Check sheet for the modelled part. Datum: model origin and axes. Units: mm. Give positions to 0.01 mm unless a question says otherwise; leave off trailing zeros. Loops run counter-clockwise (first coordinate to the right, second up) from the corner with the lowest first, then second, coordinate; pieces in that order, holes last. Notation, with made-up numbers: (-22.75, -7) - (23.25, -7) arc R25 ccw to (23.25, 7) - close; hole circle Ø7 at (28, 50). An arc over 180 degrees is marked (long way). Use CSV: the item, a comma, the result in double quotes.
from build123d import *

# Parameters (mm, degrees)
SKETCH1_R           = 0.75
SKETCH1_R_2         = 1.64
BOSS_EXTRUDE1_DEPTH = 2.3


with BuildPart() as part:
    # Sketch1 → Boss-Extrude1 (new body)
    with BuildSketch(Plane.XY):
        with BuildLine():
            Line((-16.1, -2.500431312), (-4.640508927, -3.959252063))
            ThreePointArc((-4.640508927, -3.959252063), (0, -6.1), (4.640508927, -3.959252063))
            Line((4.640508927, -3.959252063), (16.1, -2.500431312))
            ThreePointArc((16.1, -2.500431312), (18.598607316, 0.095489412), (15.90916049, 2.493137988))
            Line((15.90916049, 2.493137988), (4.649322288, 3.948898867))
            ThreePointArc((4.649322288, 3.948898867), (0, 6.1), (-4.649322288, 3.948898867))
            Line((-4.649322288, 3.948898867), (-15.90916049, 2.493137988))
            ThreePointArc((-15.90916049, 2.493137988), (-18.598607316, 0.095489412), (-16.1, -2.500431312))
        make_face()
        with Locations((-16.1, 0)):
            Circle(SKETCH1_R, mode=Mode.SUBTRACT)
        with BuildLine():
            ThreePointArc((-12.55, 0), (-13.3, -0.75), (-14.05, 0))
            ThreePointArc((-14.05, 0), (-13.3, 0.75), (-12.55, 0))
        make_face(mode=Mode.SUBTRACT)
        with BuildLine():
            ThreePointArc((-9.75, 0), (-10.5, -0.75), (-11.25, 0))
            ThreePointArc((-11.25, 0), (-10.5, 0.75), (-9.75, 0))
        make_face(mode=Mode.SUBTRACT)
        with BuildLine():
            ThreePointArc((-6.95, 0), (-7.7, -0.75), (-8.45, 0))
            ThreePointArc((-8.45, 0), (-7.7, 0.75), (-6.95, 0))
        make_face(mode=Mode.SUBTRACT)
        Circle(SKETCH1_R_2, mode=Mode.SUBTRACT)
        with BuildLine():
            ThreePointArc((8.45, 0), (7.7, -0.75), (6.95, 0))
            ThreePointArc((6.95, 0), (7.7, 0.75), (8.45, 0))
        make_face(mode=Mode.SUBTRACT)
        with BuildLine():
            ThreePointArc((11.25, 0), (10.5, -0.75), (9.75, 0))
            ThreePointArc((9.75, 0), (10.5, 0.75), (11.25, 0))
        make_face(mode=Mode.SUBTRACT)
        with BuildLine():
            ThreePointArc((14.05, 0), (13.3, -0.75), (12.55, 0))
            ThreePointArc((12.55, 0), (13.3, 0.75), (14.05, 0))
        make_face(mode=Mode.SUBTRACT)
        with Locations((16.1, 0)):
            Circle(SKETCH1_R, mode=Mode.SUBTRACT)
    extrude(amount=BOSS_EXTRUDE1_DEPTH)


solid = part.part
1. Sectioned sample at A-A, the plane x = -10.5. Record the boundary of the cut face in (y, z), and give its area (3 significant figures).
Completed:
outline,"(-3.21, 0) - (-0.75, 0) - (-0.75, 2.3) - (-3.21, 2.3) - close; (0.75, 0) - (3.19, 0) - (3.19, 2.3) - (0.75, 2.3) - close"
area,"11.3 mm²"
2. Sectioned sample at D-D, the plane x = 13.3. Record the boundary of the cut face in (y, z), and give its area (3 significant figures).
Completed:
outline,"(-2.86, 0) - (-0.75, 0) - (-0.75, 2.3) - (-2.86, 2.3) - close; (0.75, 0) - (2.83, 0) - (2.83, 2.3) - (0.75, 2.3) - close"
area,"9.63 mm²"
3. Go/stop test with flat-tipped pins: pin 1 Ø1.2 at (x, y) = (-7.7, 0) entering from +Z; pin 2 Ø1 at (y, z) = (4.5, 2) entering from -X. Record where each tip stops, or that it passes through.
Completed:
pin 1,"passes through"
pin 2,"stops at x = -4.61"
4. Sectioned sample at B-B, the plane z = 1.25. State how many separate pieces and enclosed holes the cut face has, and give its area (3 significant figures).
Completed:
separate pieces,"1"
enclosed holes,"9"
area,"246 mm²"
5. Release check for a two-part mould opening along X. For faces 1 (the face through (0, -3, 0)), 2 (the face through (-10.2, 3.23, 1.13)), 3 (the face through (-0.1, -6.1, 1.1)), 4 (the face through (-9.75, 0.03, 1.13)) record: released by +X, released by -X, zero draft, split by the parting line, or undercut.
Completed:
face 1,"zero draft"
face 2,"released by -X"
face 3,"split by the parting line"
face 4,"undercut"
6. Scan lines: line 1 along Y through (x, z) = (16.1, 1.8); line 2 along Y through (x, z) = (11, 1.75); line 3 along X through (y, z) = (-1.25, 1.1). Record each from-to range of solid material in increasing order.
Completed:
line 1,"y = -2.5 to -0.75, 0.75 to 2.5"
line 2,"y = -3.15 to -0.56, 0.56 to 3.13"
line 3,"x = -18.27 to -1.06, 1.06 to 18.27"
